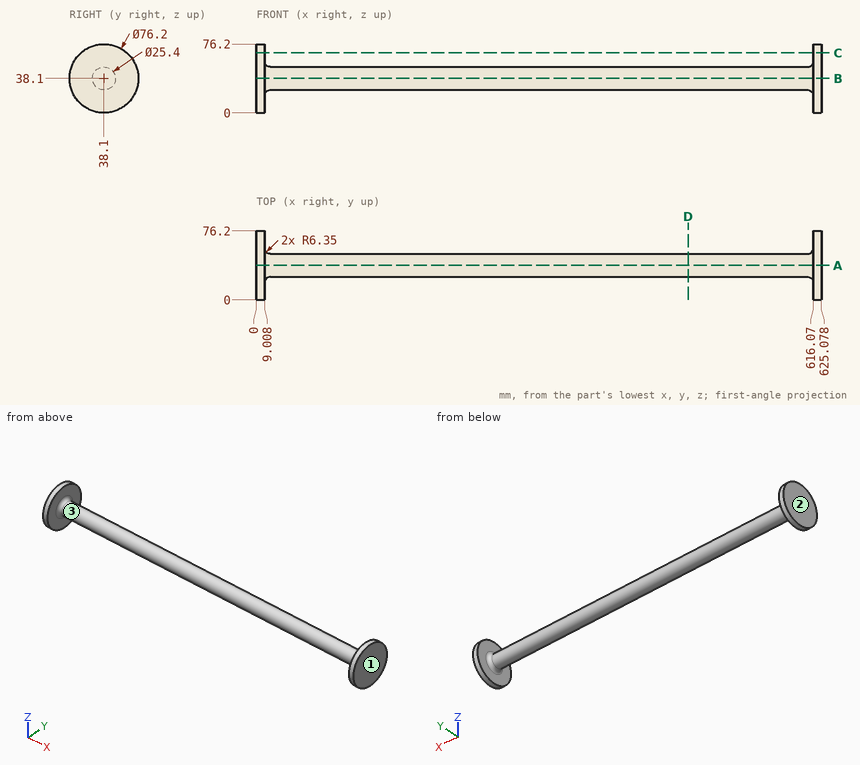
Could you check a few things on this drawing? It's one solid part, dimensions in mm from its lowest x, y, z. Give positions to 0.01 mm unless a question says otherwise; leave off trailing zeros. Order: outer loops, then holes, each group sorted by start corner. A loop starts at its lowest first (then second) coordinate and runs counter-clockwise, first axis right, second up. Notation, with made-up numbers: M 14.5,-26 L 65.5,-26 A20 cw 65.5,2 Z; hole C 60,69 d7. An arc over 180 degrees is marked long. Use one line per item in the form item = value. Start each with the question number.
Item 1: If we section it at C-C (z = 66.5): Write out the boundary of the cut face in (x, y).
Item 2: We'd pull the mould along X, two halves only. Please class the marked faces 1, 2 and 3: +X half, -X half, draft (parallel to the pull), parting line (faces both ways), or undercut.
Item 3: If I drill on line 1 along X through (y, z) = (4, 36); line 2 along X through (y, z) = (53, 48) (1 decimal); line 3 along Z through (x, y) = (61.5, 31), over which ranges is the centre line in solid material (lowest first)?
Item 4: If we section it at A-A (y = 38.1): Write out the boundary of the cut face in (x, z), then the cut area to 3 significant figures.
Item 5: Will this pin go through, and if not, where does the flat tip stop? pin 1 Ø4 at (x, y) = (85.5, 45) entering from -Z.
Item 6: If we section it at D-D (x = 477.5): Write out the boundary of the cut face in (y, z), then the cut area to 3 significant figures.
Outcome:
q1.outline = M 0,12.7 L 9.01,12.7 L 9.01,63.5 L 0,63.5 Z; M 616.07,12.7 L 625.08,12.7 L 625.08,63.5 L 616.07,63.5 Z
q2.face_1 = +X half
q2.face_2 = -X half
q2.face_3 = undercut
q3.line_1 = 0 to 9.01, 616.07 to 625.08
q3.line_2 = 0 to 9.1, 616 to 625.1
q3.line_3 = 27.57 to 48.63
q4.outline = M 0,0 L 9.01,0 L 9.01,19.05 A6.35 cw 15.36,25.4 L 609.72,25.4 A6.35 cw 616.07,19.05 L 616.07,0 L 625.08,0 L 625.08,76.2 L 616.07,76.2 L 616.07,57.15 A6.35 cw 609.72,50.8 L 15.36,50.8 A6.35 cw 9.01,57.15 L 9.01,76.2 L 0,76.2 Z
q4.area = 16,800 mm2
q5.pin_1 = 26.38
q6.outline = C 38.1,38.1 d25.4
q6.area = 507 mm2
